from build123d import *

# Parameters (mm, degrees)
F1_DEPTH = 12.7


with BuildPart() as f1:
    # F0 (on Front) → F1 (new body)
    with BuildSketch(Plane.XZ):
        Polygon((36.7118305086, 29.2767078878), (32.7487252653, 38.2864065468), (26.8258066759, 39.8544200468), (32.3351986213, 32.527134341), align=None)
        Polygon((44.6137633316, 23.4081194068), (36.7118305086, 29.2767078878), (39.4362804042, 23.0829605448), (44.8738240342, 15.8512304175), align=None)
        Polygon((39.4362804042, 23.0829605448), (36.7118305086, 29.2767078878), (32.3351986213, 32.527134341), align=None)
        Polygon((32.3351986213, 32.527134341), (26.8258066759, 39.8544200468), (20.0559669896, 41.6466445828), align=None)
        Polygon((20.0559669896, 41.6466445828), (26.8258066759, 39.8544200468), (23.143676418, 44.7515158919), (15.5853806795, 44.9668488809), align=None)
        Polygon((44.8738240342, 15.8512304175), (39.4362804042, 23.0829605448), (45.0653487584, 10.2858717752), align=None)
        Polygon((6.5411333928, 45.2245160678), (20.0559669896, 41.6466445828), (15.5853806795, 44.9668488809), align=None)
        Polygon((44.8738240342, 15.8512304175), (45.0653487584, 10.2858717752), (47.8850571971, 3.8755642564), (49.4179902366, 9.8076589327), align=None)
        Polygon((47.8850571971, 3.8755642564), (45.0653487584, 10.2858717752), (45.5914042437, -5.0003397286), align=None)
        Polygon((-5.2700710808, 45.5610128193), (6.5411333928, 45.2245160678), (0, 46.9561936707), align=None)
        Polygon((0, 46.9561936707), (6.5411333928, 45.2245160678), (15.5853806795, 44.9668488809), (9.5150217621, 49.4751684548), align=None)
        Polygon((50.3520142156, -1.7328003913), (47.8850571971, 3.8755642564), (45.5914042437, -5.0003397286), (45.7789038594, -10.4487360706), align=None)
        Polygon((45.7789038594, -10.4487360706), (45.5914042437, -5.0003397286), (42.6351039178, -16.440535075), align=None)
        Polygon((-5.2700710808, 45.5610128193), (0, 46.9561936707), (-9.5150217621, 49.4751684548), (-14.433823419, 45.82208466), align=None)
        Polygon((-20.0559669896, 41.6466445828), (-5.2700710808, 45.5610128193), (-14.433823419, 45.82208466), align=None)
        Polygon((46.1174311574, -20.2857209931), (45.7789038594, -10.4487360706), (42.6351039178, -16.440535075), (40.371362632, -25.2006878565), align=None)
        Polygon((40.371362632, -25.2006878565), (42.6351039178, -16.440535075), (36.1396037465, -28.8203722726), align=None)
        Polygon((-25.4391722107, 40.2215129805), (-20.0559669896, 41.6466445828), (-14.433823419, 45.82208466), (-20.5582977883, 45.99656862), align=None)
        Polygon((-31.2796204782, 33.3110885798), (-20.0559669896, 41.6466445828), (-25.4391722107, 40.2215129805), align=None)
        Polygon((40.371362632, -25.2006878565), (36.1396037465, -28.8203722726), (32.8858829718, -35.0216704662), (38.4795494638, -32.5215652427), align=None)
        Polygon((32.8858829718, -35.0216704662), (36.1396037465, -28.8203722726), (24.5163525755, -38.7624559943), align=None)
        Polygon((-38.9068697692, 24.2865193693), (-31.2796204782, 33.3110885798), (-36.7118305086, 29.2767078878), align=None)
        Polygon((-36.7118305086, 29.2767078878), (-31.2796204782, 33.3110885798), (-25.4391722107, 40.2215129805), (-32.7487252653, 38.2864065468), align=None)
        Polygon((30.0392094677, -40.4471732921), (32.8858829718, -35.0216704662), (24.5163525755, -38.7624559943), (20.3735288846, -42.3060686525), align=None)
        Polygon((20.3735288846, -42.3060686525), (24.5163525755, -38.7624559943), (13.7288245836, -43.5839724576), align=None)
        Polygon((-38.9068697692, 24.2865193693), (-36.7118305086, 29.2767078878), (-44.6137633316, 23.4081194068), (-44.8244900831, 17.284784924), align=None)
        Polygon((-45.0653487584, 10.2858717752), (-38.9068697692, 24.2865193693), (-44.8244900831, 17.284784924), align=None)
        Polygon((12.8937326976, -48.703999732), (20.3735288846, -42.3060686525), (13.7288245836, -43.5839724576), (5.4684417421, -47.2759741742), align=None)
        Polygon((5.4684417421, -47.2759741742), (13.7288245836, -43.5839724576), (0, -46.2242881707), align=None)
        Polygon((-47.3075095617, 5.1885574364), (-45.0653487584, 10.2858717752), (-44.8244900831, 17.284784924), (-48.7794544472, 12.6052670182), align=None)
        Polygon((-45.5461821411, -3.6862680312), (-45.0653487584, 10.2858717752), (-47.3075095617, 5.1885574364), align=None)
        Polygon((5.4684417421, -47.2759741742), (0, -46.2242881707), (-6.8770318811, -47.5468730158), (-1.4347768951, -50.3613874713), align=None)
        Polygon((-6.8770318811, -47.5468730158), (0, -46.2242881707), (-15.0200126245, -43.3356522862), align=None)
        Polygon((-43.2460019659, -15.2762185204), (-45.5461821411, -3.6862680312), (-45.7789038594, -10.4487360706), align=None)
        Polygon((-45.7789038594, -10.4487360706), (-45.5461821411, -3.6862680312), (-47.3075095617, 5.1885574364), (-50.3520142156, -1.7328003913), align=None)
        Polygon((-12.8937326976, -48.703999732), (-6.8770318811, -47.5468730158), (-15.0200126245, -43.3356522862), (-20.3735288846, -42.3060686525), align=None)
        Polygon((-20.3735288846, -42.3060686525), (-15.0200126245, -43.3356522862), (-25.515539679, -37.9077896286), align=None)
        Polygon((-43.2460019659, -15.2762185204), (-45.7789038594, -10.4487360706), (-46.1174311574, -20.2857209931), (-41.4614014616, -24.2683104051), align=None)
        Polygon((-36.1396037465, -28.8203722726), (-43.2460019659, -15.2762185204), (-41.4614014616, -24.2683104051), align=None)
        Polygon((-30.0392094677, -40.4471732921), (-20.3735288846, -42.3060686525), (-25.515539679, -37.9077896286), (-33.5523273154, -33.7514876846), align=None)
        Polygon((-33.5523273154, -33.7514876846), (-25.515539679, -37.9077896286), (-36.1396037465, -28.8203722726), align=None)
        Polygon((-33.5523273154, -33.7514876846), (-36.1396037465, -28.8203722726), (-41.4614014616, -24.2683104051), (-40.2686869878, -30.2780577489), align=None)
    extrude(amount=F1_DEPTH)


solid = f1.part
Can you work these out from the model? Positions are in its coordinate system, mm. A direction names the side the tool comes from. Coordinates: 2 decimals unless noted, no trailing zeros. Order: outer loops, then holes, each group sorted by start corner. A loop starts at its lowest first (then second) coordinate and runs counter-clockwise, first axis right, second up. Notation, with made-up numbers: (-31.75, -7.75) -> (17.25, -7.75) arc R23 ccw to (17.25, 30.25) -> close; hole circle Ø1 at (87.5, 12.5). An arc over 180 degrees is marked (long way). Use one line per item in the form item = value.
Q1. Imagine slicing it at A-A, the plane z = -14. List the corners of the cut face in (x, y) for me.
From the geometry:
outline = (-45.9, -12.7) -> (-43.5, -12.7) -> (-43.5, 0) -> (-45.9, 0) -> close; (43.27, -12.7) -> (45.9, -12.7) -> (45.9, 0) -> (43.27, 0) -> close
Q2. Will these pins go through, and if not, where does the flat tip stop? P1, Ø2, axis at y = -3, z = 5.5, coming from the -X side; P2, Ø1.5, axis at x = -32.5, y = -11.5, coming from the -Z side; P3, Ø2, axis at x = -25, y = -7, coming from the -Z side.
From the geometry:
P1 = -47.61
P2 = -37.19
P3 = -41.61
Q3. We'd pull the mould along X, two halves only. Please class faces 1 (the face through (19.2, -6.26, -41.14)), 2 (the face through (-25.274, -6.261, -41.364)), 3 (the face through (48.64, -6.26, 6.8)): released by +X, released by -X, zero draft, split by the parting line, or undercut.
From the geometry:
face_1 = undercut
face_2 = released by -X
face_3 = released by +X
Q4. Which directions (+Z, -Z, +X, -X, +Y, -Y) give clear straight access to the entire face, cutting with the end or side of a thin tool? Please do faces 4 (the face through (-48.054, -6.261, 8.949)), 5 (the face through (9.13, -6.26, -47.98)), 6 (the face through (-30.75, -6.26, -33.43)), 7 (the face through (4.824, -6.261, 48.233)), 8 (the face through (11, -12.7, 44.2)).
From the geometry:
face_4 = -X, +Y, -Y
face_5 = -Z, +Y, -Y
face_6 = +Y, -Y
face_7 = +Z, +Y, -Y
face_8 = +Z, -Z, +X, -X, -Y
Q5. Imagine slicing it at B-B, the plane x = -27.5. List the corners of the cut face in (y, z) for me.
From the geometry:
outline = (-12.7, -40.94) -> (0, -40.94) -> (0, -36.21) -> (-12.7, -36.21) -> close; (-12.7, 36.12) -> (0, 36.12) -> (0, 39.68) -> (-12.7, 39.68) -> close
Q6. I need wall thicknesses on L1, parallel to Z at x = 32, y = -2.5; L2, parallel to X at y = -10.5, z = -28.5; L3, parallel to X at y = -7.25, z = -30. Which ranges of each line are inside material? Lowest first, please.
From the geometry:
L1 = -36.71 to -32.36, 32.78 to 38.48
L2 = -40.62 to -36.31, 36.31 to 39.52
L3 = -40.32 to -34.76, 34.76 to 39.13
